CAD build for the part. Positions are in the model's coordinates, mm. Face numbers are marked on the shaded views. A direction names the side the tool comes from. Give positions to 0.01 mm unless a question says otherwise; leave off trailing zeros. Write each loop counter-clockwise with the first axis right and the second up, starting at its lowest first coordinate (ties: lowest second). Pieces come first, ordered by that corner, then holes. Notation, with made-up numbers: (85.25, -37.75) - (107.25, -37.75) arc R7 ccw to (107.25, -32.75) - close; hole circle Ø8 at (45, 53.5). An arc over 180 degrees is marked (long way). Answer as a JSON object with one key per item and string values.
from build123d import *

# Parameters (mm, degrees)
F0_W            = 9.2476086318
F0_H            = 25
F1_DEPTH        = 20
F3_D            = 8.8
F3_DEPTH        = 40.701
F4_D            = 9
F4_DEPTH        = 37.301
F6_D            = 10.5
F7_R            = 5
F8_SIZE         = 1
F10_D           = 8
F10_CBORE_D     = 17
F10_CBORE_DEPTH = 8


# Not quite as in the source:
# - a feature names something its author has since deleted; it is built from what else it names


with BuildPart() as f1:
    # F0 (on Top) → F1 (new body)
    with BuildSketch(Plane.XY):
        with BuildLine():
            ThreePointArc((21.4269106499, -2.3), (-21.55, 0), (21.4269106499, 2.3))
            Line((21.4269106499, 2.3), (40, 2.3))
            Line((40, 2.3), (40, 27.2765494883))
            Line((40, 27.2765494883), (21.9314807528, 27.2765494883))
            ThreePointArc((21.9314807528, 27.2765494883), (-15.122800231, 31.5642347155), (-35, 0))
            ThreePointArc((-35, 0), (-1.1506219411, -34.9810815892), (34.9243468085, -2.3))
            Line((34.9243468085, -2.3), (21.4269106499, -2.3))
        make_face()
        with BuildLine():
            Line((40, -2.3), (34.9243468085, -2.3))
            ThreePointArc((34.9243468085, -2.3), (-1.1506219411, -34.9810815892), (-35, 0))
            Line((-35, 0), (-35, -25))
            Line((-35, -25), (-44.2476086318, -25))
            Line((-44.2476086318, -25), (-70, -25))
            Line((-70, -25), (-70, -43))
            Line((-70, -43), (70, -43))
            Line((70, -43), (70, -25))
            Line((70, -25), (40, -25))
            Line((40, -25), (40, -2.3))
        make_face()
        with Locations((-39.6238043159, -12.5)):
            Rectangle(F0_W, F0_H)
    extrude(amount=F1_DEPTH)

    # F3 (through all, one way)
    with BuildSketch(Plane(origin=(0, -2.3, 0), x_dir=(-1, 0, 0), z_dir=(0, 1, 0))):
        with Locations((-32, 10)):
            Circle(F3_D / 2)
    extrude(amount=-F3_DEPTH, mode=Mode.SUBTRACT)

    # F4 (through all, one way)
    with BuildSketch(Plane(origin=(0, -2.3, 0), x_dir=(-1, 0, 0), z_dir=(0, -1, 0))):
        with Locations((-32, -10)):
            Circle(F4_D / 2)
    extrude(amount=-F4_DEPTH, mode=Mode.SUBTRACT)

    # F6 (through all)
    with Locations(Plane(origin=(0, -25, 0), x_dir=(-1, 0, 0), z_dir=(0, 1, 0))):
        with Locations((55, 10), (-55, 10)):
            Hole(F6_D / 2)

    # F7
    f7_edges = [f1.edges().sort_by_distance(p)[0] for p in [
        (40, -25, 10),
        (21.931481, 27.276549, 10),
        (-44.247609, -25, 10),
        (-70, -25, 10),
    ]]
    fillet(f7_edges, radius=F7_R)

    # F8
    f8_edges = [f1.edges().sort_by_distance(p)[0] for p in [
        (31.813386, 27.276549, 20),
        (22.073202, 27.524032, 20),
        (40, 14.788275, 20),
        (-15.833984, 31.213538, 20),
        (30.713455, 2.3, 20),
        (-39.623804, 0, 20),
        (-21.55, 0, 20),
        (-44.247609, -10, 20),
        (30.713455, -2.3, 20),
        (-45.712075, -23.535534, 20),
        (40, -11.15, 20),
        (-57.123804, -25, 20),
        (41.464466, -23.535534, 20),
        (-68.535534, -26.464466, 20),
        (57.5, -25, 20),
        (-70, -36.5, 20),
        (70, -34, 20),
        (0, -43, 20),
        (31.813386, 27.276549, 0),
        (22.073202, 27.524032, 0),
        (40, 14.788275, 0),
        (-15.833984, 31.213538, 0),
        (30.713455, 2.3, 0),
        (-39.623804, 0, 0),
        (-21.55, 0, 0),
        (-44.247609, -10, 0),
        (30.713455, -2.3, 0),
        (-45.712075, -23.535534, 0),
        (40, -11.15, 0),
        (-57.123804, -25, 0),
        (41.464466, -23.535534, 0),
        (-68.535534, -26.464466, 0),
        (57.5, -25, 0),
        (-70, -36.5, 0),
        (70, -34, 0),
        (0, -43, 0),
        (23.626772, 27.276549, 10),
        (40, 27.276549, 10),
        (36.5, 27.276549, 10),
        (-70, -30, 10),
        (-70, -43, 10),
        (70, -43, 10),
        (70, -25, 10),
    ]]
    chamfer(f8_edges, length=F8_SIZE)

    # F10 (through all)
    with Locations(Plane.XY.offset(20)):
        with Locations((-20, -30), (20, -30)):
            CounterBoreHole(F10_D / 2, F10_CBORE_D / 2, F10_CBORE_DEPTH)


solid = f1.part
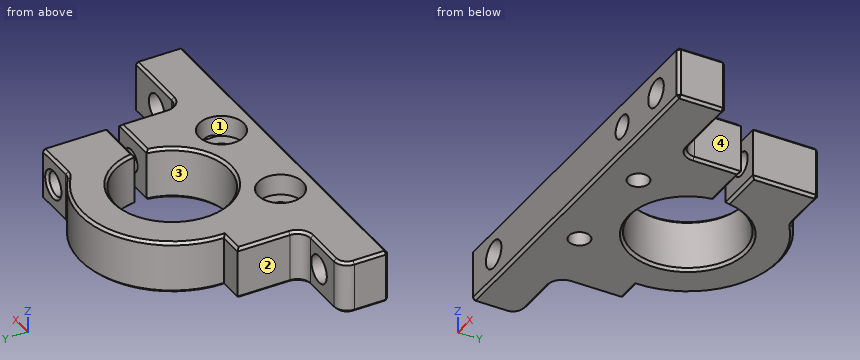
Item 1: Cut at B-B (x = 0). Give the cut face in (y, z), and give its area (3 significant figures).
Entries:
{"outline": "(-43, 1) - (-42, 0) - (-22.55, 0) - (-21.55, 1) - (-21.55, 19) - (-22.55, 20) - (-42, 20) - (-43, 19) - close; (21.55, 1) - (22.55, 0) - (34, 0) - (35, 1) - (35, 19) - (34, 20) - (22.55, 20) - (21.55, 19) - close", "area": "694 mm2"}
Item 2: Probe line 1 (Z direction, x = -55, y = -32.5); line 2 (Y direction, x = 38, z = 17.5); line 3 (X direction, y = 14, z = 10). List the from-to ranges inside material, lowest first. Write a range as from..to.
Entries:
{"line 1": "0..4.75, 15.25..20", "line 2": "-43..-2.3, 2.3..27.28", "line 3": "-32.08..-16.38, 16.38..27.5, 36.5..40"}
Item 3: Cut at D-D (x = -55). Give the cut face in (y, z).
Entries:
{"outline": "(-43, 1) - (-42, 0) - (-26, 0) - (-25, 1) - (-25, 4.75) - (-43, 4.75) - close; (-43, 15.25) - (-25, 15.25) - (-25, 19) - (-26, 20) - (-42, 20) - (-43, 19) - close"}
Item 4: Cut at C-C (y = -11.5). State how many separate pieces and enclosed holes the cut face has, and give its area (3 significant figures).
Entries:
{"separate pieces": "2", "enclosed holes": "1", "area": "891 mm2"}
Item 5: Flat gauge pins, fed straight in: P1, Ø1.5, axis at y = -23.5, z = 13.5, coming from the -X side; P2, Ø2, axis at y = 23, z = 8, coming from the -X side; P3, Ø9, axis at y = -9, z = 10.5, coming from the +X side; P4, Ø8.5, axis at x = 55, z = 10, coming from the -Y side. Where does each tip first touch, or does it go through?
Entries:
{"P1": "x = -46.61", "P2": "x = -27.22", "P3": "x = 40", "P4": "through"}
Item 6: Which spindle directions (+Z, -Z, +X, -X, +Y, -Y) get a long thin tool onto all of the face, cutting with end or side? Do the marked faces 1, 2, 3 and 4. Say none if no direction does.
Entries:
{"face 1": "+Z", "face 2": "+Z, -Z, -X, +Y", "face 3": "+Z, -Z", "face 4": "+Z, -Z, +X, +Y"}
Item 7: Cut at A-A (x = 32). Give the cut face in (y, z).
Entries:
{"outline": "(-43, 1) - (-42, 0) - (-3.3, 0) - (-2.3, 1) - (-2.3, 5.6) - (-43, 5.6) - close; (-43, 14.4) - (-2.3, 14.4) - (-2.3, 19) - (-3.3, 20) - (-42, 20) - (-43, 19) - close; (2.3, 1) - (3.3, 0) - (26.28, 0) - (27.28, 1) - (27.28, 4.5) - (26.28, 5.5) - (2.3, 5.5) - close; (2.3, 14.5) - (26.28, 14.5) - (27.28, 15.5) - (27.28, 19) - (26.28, 20) - (3.3, 20) - (2.3, 19) - close"}
